```python
from build123d import *

# Parameters (mm, degrees)
BOSS_EXTRUDE1_DEPTH = 5
BOSS_EXTRUDE2_DEPTH = 2
FILLET1_R           = 5
FILLET2_R           = 1
FILLET3_R           = 1


with BuildPart() as part:
    # Sketch32 → Boss-Extrude1 (new body)
    with BuildSketch(Plane(origin=(0, 0, 0), x_dir=(0, 0, -1), z_dir=(1, 0, 0))):
        Polygon((-23.663373299, 32.245792092), (-0.6, 4.759934105), (-0.6, 58.641752364), align=None)
    extrude(amount=-BOSS_EXTRUDE1_DEPTH)

    # Sketch33 → Boss-Extrude2 (add)
    with BuildSketch(Plane(origin=(0, 0, 0), x_dir=(0, 0, -1), z_dir=(1, 0, 0))):
        Polygon((0, 0), (2, 0), (2, 63.28), (0, 63.28), (-27.086136094, 32.28), align=None)
    extrude(amount=BOSS_EXTRUDE2_DEPTH)

    # Fillet1
    fillet1_edges = [part.edges().sort_by_distance(p)[0] for p in [
        (1, 32.28, 27.086136094),
    ]]
    fillet(fillet1_edges, radius=FILLET1_R)

    # Fillet2
    fillet2_edges = [part.edges().sort_by_distance(p)[0] for p in [
        (-2.5, 32.245792092, 23.663373299),
        (-2.5, 58.641752364, 0.6),
        (-2.5, 4.759934105, 0.6),
    ]]
    fillet(fillet2_edges, radius=FILLET2_R)

    # Fillet3
    fillet3_edges = [part.edges().sort_by_distance(p)[0] for p in [
        (1, 0, 0),
        (1, 0, -2),
        (1, 63.28, -2),
        (1, 63.28, 0),
    ]]
    fillet(fillet3_edges, radius=FILLET3_R)


solid = part.part
```
For this review, take the finished solid that the model builds, in its own axes (mm). A direction names the side the tool comes from. Round coordinates to 2 decimals unless told otherwise and drop trailing zeros. Write each loop counter-clockwise with the first axis right and the second up, starting at its lowest first coordinate (ties: lowest second). Pieces come first, ordered by that corner, then holes. Notation, with made-up numbers: (43.5, 46.5) - (59.5, 46.5) arc R17 ccw to (59.5, 70.5) - close; hole circle Ø3 at (25, -23.5). An arc over 180 degrees is marked (long way). Write each question's results on one line, items separated by ' | '.
Item 1: Take a section at C-C on z = 16. State the section outline as (x, y) points.
Calculated:
outline: (-5, 23.11) - (0, 23.11) - (0, 19.07) - (2, 19.07) - (2, 44.97) - (0, 44.97) - (0, 41.02) - (-5, 41.02) - close
Item 2: For pin 1 (5 mm diameter, centred on y = 9.5, z = 14, fed in from +X); pin 2 (2 mm diameter, centred on x = 0.5, z = 3.5, fed in from -Y); pin 3 (4 mm diameter, centred on x = -3.5, y = 38.5, fed in from -Z); pin 4 (1.5 mm diameter, centred on x = -1.5, z = 14, fed in from -Y), all flat-tipped, find the tip position at first contact; note any pin that passes through.
Calculated:
pin 1: passes through | pin 2: stops at y = 2.98 | pin 3: stops at z = 0.6 | pin 4: stops at y = 19.84
Item 3: Take a section at B-B on y = 12. State the section outline as (x, z) points, then the cut area to 3 significant figures.
Calculated:
outline: (-5, 0.6) - (0, 0.6) - (0, -2) - (2, -2) - (2, 10.07) - (0, 10.07) - (0, 6.68) - (-5, 6.68) - close | area: 54.5 mm^2
Item 4: Take a section at A-A on x = 0.75. State the section outline as (y, z) points, then the cut area to 3 significant figures.
Calculated:
outline: (0, -1) arc R1 ccw to (1, -2) - (62.28, -2) arc R1 ccw to (63.28, -1) - (63.28, -0.45) arc R1 ccw to (62.94, 0.3) - (35.5, 24.27) arc R5 ccw to (29, 24.33) - (0.36, 0.3) arc R1 ccw to (0, -0.47) - close | area: 979 mm^2
Item 5: To check wall thickness, follow line 1 along X through (y, z) = (58.5, -1); line 2 along Y through (x, z) = (-0.5, 22.75); line 3 along Z through (x, y) = (-1.5, 53). State the ranges of each line that lie inside material, in increasing order. Write a range as from..to.
Calculated:
line 1: x = 0..2 | line 2: y = 31.16..33.29 | line 3: z = 0.6..5.53
Item 6: For faces 1 (the face through (-2.535, 56.908, 1.233)), 2 (the face through (0, 32, 0)), 3 (the face through (-2.535, 32.233, 23.347)), 4 (the face through (-2.535, 6.562, 1.274)), 5 (the face through (-2.46, 44.93, 12.58)), list the 3-axis set-ups (+Z, -Z, +X, -X, +Y, -Y) from which the entire face can be reached by the end or side of a thin tool; tool diameter is ignored.
Calculated:
face 1: -X, +Y | face 2: -X | face 3: +Z, -X | face 4: -X, -Y | face 5: +Z, -X, +Y
Item 7: Take a section at D-D on x = -2.5. State the section outline as (y, z) points, then the cut area to 3 significant figures.
Calculated:
outline: (6.86, 2.37) arc R1 ccw to (7.51, 0.6) - (55.98, 0.6) arc R1 ccw to (56.64, 2.35) - (32.89, 23.1) arc R1 ccw to (31.59, 23.11) - close | area: 618 mm^2
